The model under review builds one solid part; all positions refer to its coordinate system, in mm. A direction names the side the tool comes from. Give positions to 0.01 mm unless a question says otherwise; leave off trailing zeros. Order: outer loops, then holes, each group sorted by start corner. A loop starts at its lowest first (then second) coordinate and runs counter-clockwise, first axis right, second up. Notation, with made-up numbers: (35, 20.5) - (72, 20.5) arc R21 cw to (72, 36.5) - close; hole circle Ø3 at (-33.75, 65.5). An arc over 180 degrees is marked (long way). Use CSV: the item, a comma, the result in double quotes. Start each with the question number.
1. Take a section at A-A, the plane z = -19. Count the separate pieces of the cut face and the enclosed holes in it, then the cut area to 3 significant figures.
2. For pin 1 (2.5 mm diameter, centred on x = 1.5, y = 16, fed in from -Z); pin 2 (1.5 mm diameter, centred on x = 1.5, y = 48.5, fed in from -Z); pin 3 (1 mm diameter, centred on y = 69.5, z = -6.5, fed in from -X); pin 4 (2 mm diameter, centred on x = 2, z = -20, fed in from +Y), all flat-tipped, find the tip position at first contact; note any pin that passes through.
3. To check wall thickness, follow line 1 (Z direction, x = 3.15, y = 46); line 2 (X direction, y = 51.5, z = -15); line 3 (X direction, y = 23.5, z = -16). State the ranges of each line that lie inside material, in increasing order. Write a range as [from, to].
4. Take a section at B-B, the plane y = 36.5. State the section outline as (x, z) points, then the cut area to 3 significant figures.
5. Machinability: for faces 4 (the cylindrical face through (3.04, 50.56, -12.32)), 5 (the flat face through (3, 63, -25)), which of the approach directions +Z, -Z, +X, -X, +Y, -Y give a long, thin tool a straight path to every point of the face, cutting with its end or side? Answer none if there is none.
6. Draft analysis for pull direction Y (two halves, no side actions). For faces 1 (the flat face through (3, 13, -25)), 2 (the cylindrical face through (3.04, 10.56, -12.32)), 3 (the flat face through (2, 0, 10)), state which applies: released by +Y, released by -Y, zero draft, split by the parting line, or undercut.
```python
from build123d import *

# Parameters (mm, degrees)
SKETCH1_W           = 90
SKETCH1_H           = 20
BOSS_EXTRUDE1_DEPTH = 5
SKETCH2_R           = 2.5
BOSS_EXTRUDE2_DEPTH = 25


with BuildPart() as part:
    # Sketch1 → Boss-Extrude1 (new body)
    with BuildSketch(Plane.YZ):
        with Locations((45, 10)):
            Rectangle(SKETCH1_W, SKETCH1_H)
    extrude(amount=BOSS_EXTRUDE1_DEPTH)

    # Sketch2 → Boss-Extrude2 (add)
    with BuildSketch(Plane(origin=(0, 0, 0), x_dir=(1, 0, 0), z_dir=(0, 0, -1))):
        with Locations(Location((2.5, -3, 0), (0, 0, 180))):
            Circle(SKETCH2_R)
        with Locations(Location((2.5, -13, 0), (0, 0, 180))):
            Circle(SKETCH2_R)
        with Locations(Location((2.5, -23, 0), (0, 0, 180))):
            Circle(SKETCH2_R)
        with Locations(Location((2.5, -33, 0), (0, 0, 180))):
            Circle(SKETCH2_R)
        with Locations(Location((2.5, -43, 0), (0, 0, 180))):
            Circle(SKETCH2_R)
        with Locations(Location((2.5, -53, 0), (0, 0, 180))):
            Circle(SKETCH2_R)
        with Locations(Location((2.5, -63, 0), (0, 0, 180))):
            Circle(SKETCH2_R)
        with Locations(Location((2.5, -73, 0), (0, 0, 180))):
            Circle(SKETCH2_R)
        with Locations(Location((2.5, -83, 0), (0, 0, 180))):
            Circle(SKETCH2_R)
    extrude(amount=BOSS_EXTRUDE2_DEPTH)


solid = part.part
```
Determined:
1,separate pieces,"9"
1,enclosed holes,"0"
1,area,"177 mm²"
2,pin 1,"stops at z = -25"
2,pin 2,"stops at z = 0"
2,pin 3,"passes through"
2,pin 4,"stops at y = 85.5"
3,line 1,"z = [0, 20]"
3,line 2,"x = [0.5, 4.5]"
3,line 3,"x = [0.05, 4.95]"
4,outline,"(0, 0) - (5, 0) - (5, 20) - (0, 20) - close"
4,area,"100 mm²"
5,face 4,"-Z"
5,face 5,"-Z, +X, -X, +Y, -Y"
6,face 1,"zero draft"
6,face 2,"undercut"
6,face 3,"released by -Y"
